Read the model definition and answer for the solid it produces. Units are mm, in the model's axes. Round coordinates to 2 decimals unless told otherwise and drop trailing zeros. Loops run counter-clockwise (first coordinate to the right, second up) from the corner with the lowest first, then second, coordinate; pieces in that order, holes last. Notation, with made-up numbers: M -28.75,-23.75 L 19.25,-23.75 A16 cw 19.25,5.25 Z; hole C -35.5,-4 d7. An arc over 180 degrees is marked long. Write each question's results on one line, items separated by ' | '.
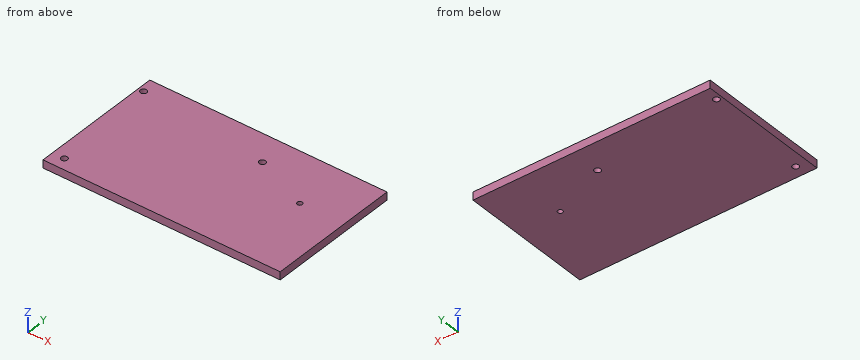
from build123d import *

# Parameters (mm, degrees)
F0_W     = 300
F0_H     = 170
F0_R     = 4
F1_DEPTH = 10
F3_D     = 6.3


with BuildPart() as f1:
    # F0 (on Top) → F1 (new body)
    with BuildSketch(Plane.XY):
        with Locations((-150, -85)):
            Rectangle(F0_W, F0_H)
        with Locations((-285, -155)):
            Circle(F0_R, mode=Mode.SUBTRACT)
        with Locations((-293.1499779224, -18.4999983758)):
            Circle(F0_R, mode=Mode.SUBTRACT)
        with Locations((-127.52, -37.86)):
            Circle(F0_R, mode=Mode.SUBTRACT)
    extrude(amount=F1_DEPTH)

    # F3 (through all)
    with Locations(Plane(origin=(0, 0, 0), x_dir=(1, 0, 0), z_dir=(0, 0, -1))):
        with Locations((-55.8166801929, 68.5865059495)):
            Hole(F3_D / 2)


solid = f1.part
Item 1: The part is cut by section A-A (x = -127.52). Determine the outline of the cut face in (y, z).
Outcome:
outline: M -170,0 L -41.86,0 L -41.86,10 L -170,10 Z; M -33.86,0 L 0,0 L 0,10 L -33.86,10 Z
Item 2: Straight lines are drawn through the part: line 1 (Y direction, x = -285, z = 5.5); line 2 (X direction, y = -153, z = 6.75). For each, find the intervals that lie inside material, in ascending order.
Outcome:
line 1: y = -170 to -159, -151 to 0 | line 2: x = -300 to -288.46, -281.54 to 0
Item 3: The part is cut by section B-B (y = -37.86). Determine the outline of the cut face in (x, z).
Outcome:
outline: M -300,0 L -131.52,0 L -131.52,10 L -300,10 Z; M -123.52,0 L 0,0 L 0,10 L -123.52,10 Z
Item 4: A flat-ended cylindrical pin translates along its axis: pin 1 (8 mm diameter, centred on x = -55.82, y = -68.59, fed in from +Z). Find the tip coordinate at first contact, or state that the pin passes through.
Outcome:
pin 1: stops at z = 10
